Here's the drawing with two shaded views (mm, measured from the low corner). I have some questions. A direction names the side the tool comes from. Round coordinates to 2 decimals unless told otherwise and drop trailing zeros. Order: outer loops, then holes, each group sorted by start corner. A loop starts at its lowest first (then second) coordinate and runs counter-clockwise, first axis right, second up. Notation, with made-up numbers: (46, -28.75) -> (86, -28.75) arc R21 ccw to (86, -10.75) -> close; hole circle Ø2 at (-33, 82.5). An arc over 180 degrees is marked (long way). Use a Markdown table: item, result. Add a question column.
Q1. I'm going to push flat-ended pins straight in: pin 1 Ø1 at (x, z) = (50.5, 120.5) entering from -Y; pin 2 Ø20.5 at (x, z) = (62.75, 138) entering from +Y; pin 3 Ø3 at (y, z) = (19, 29) entering from -X; pin 4 Ø6 at (x, y) = (134.5, 8) entering from -Z. Where does each tip first touch, or does it pass through?
Q2. I need wall thicknesses on line 1 along Z through (x, y) = (62, 9); line 2 along Z through (x, y) = (107, 4); line 3 along X through (y, z) = (14, 32). Which ranges of each line are inside material? Lowest first, please. Write a range as [from, to].
Q3. If we section it at D-D on x = 62.75: Give the number of separate pieces and of enclosed holes in the cut face, plus the area to 3 significant figures.
Q4. If we section it at B-B on x = 85: List the corners of the cut face in (y, z) for me, plus the area to 3 significant figures.
Q5. If we section it at A-A on z = 138: List the corners of the cut face in (x, y) for me, plus the area to 3 significant figures.
Q6. For the marked faces 1 and 2, which set-ups out of +Z, -Z, +X, -X, +Y, -Y let a thin tool reach every point of the face, with its end or its side?
Q7. If we section it at C-C on y = 12.5: List the corners of the cut face in (x, z) for me, plus the area to 3 significant figures.
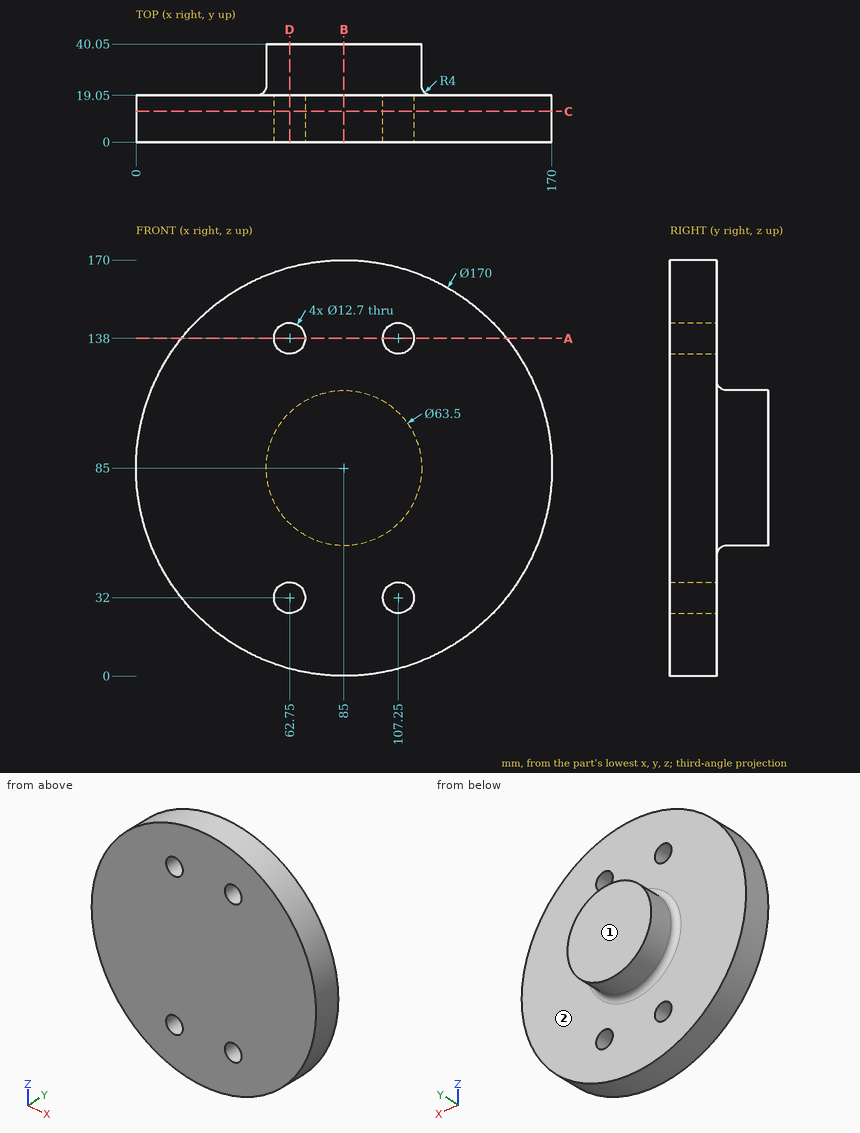
Answer below:
| question | item | result |
|---|---|---|
| 1 | pin 1 | y = 0 |
| 1 | pin 2 | y = 19.05 |
| 1 | pin 3 | x = 19.77 |
| 1 | pin 4 | z = 13.85 |
| 2 | line 1 | [3.17, 25.69], [38.31, 131.69], [144.31, 166.83] |
| 2 | line 2 | [2.9, 25.65], [38.35, 131.65], [144.35, 167.1] |
| 2 | line 3 | [18.55, 56.4], [69.1, 100.9], [113.6, 151.45] |
| 3 | separate pieces | 3 |
| 3 | enclosed holes | 0 |
| 3 | area | 3,600 mm² |
| 4 | outline | (0, 0) -> (19.05, 0) -> (19.05, 49.25) arc R4 cw to (23.05, 53.25) -> (40.05, 53.25) -> (40.05, 116.75) -> (23.05, 116.75) arc R4 cw to (19.05, 120.75) -> (19.05, 170) -> (0, 170) -> close |
| 4 | area | 4,580 mm² |
| 5 | outline | (18.55, 0) -> (56.4, 0) -> (56.4, 19.05) -> (18.55, 19.05) -> close; (69.1, 0) -> (100.9, 0) -> (100.9, 19.05) -> (69.1, 19.05) -> close; (113.6, 0) -> (151.45, 0) -> (151.45, 19.05) -> (113.6, 19.05) -> close |
| 5 | area | 2,050 mm² |
| 6 | face 1 | +Z, -Z, +X, -X, +Y |
| 6 | face 2 | +Y |
| 7 | outline | circle Ø170 at (85, 85); hole circle Ø12.7 at (62.75, 32); hole circle Ø12.7 at (62.75, 138); hole circle Ø12.7 at (107.25, 32); hole circle Ø12.7 at (107.25, 138) |
| 7 | area | 22,200 mm² |
